```python
from build123d import *

# Parameters (mm, degrees)
SKETCH068_R         = 1
PAD021_DEPTH        = 1.3
SKETCH002_R         = 0.5
POCKET_DEPTH        = 0.001
POCKET_DEPTH_BACK   = 1.301
LINEARPATTERN_COUNT = 7
LINEARPATTERN_PITCH = 2.54


with BuildPart() as part:
    # Sketch068 → Pad021 (new body)
    with BuildSketch(Plane.XY):
        Polygon((-13.25, 19.61), (13.25, 19.61), (13.89, 18.97), (13.89, -18.97), (13.25, -19.61), (-13.25, -19.61), (-13.89, -18.97), (-13.89, 18.97), align=None)
        with Locations((11.39, 17.11)):
            Circle(SKETCH068_R, mode=Mode.SUBTRACT)
        with Locations((-11.39, 17.11)):
            Circle(SKETCH068_R, mode=Mode.SUBTRACT)
        with Locations((-11.39, -17.11)):
            Circle(SKETCH068_R, mode=Mode.SUBTRACT)
        with Locations((11.39, -17.11)):
            Circle(SKETCH068_R, mode=Mode.SUBTRACT)
    extrude(amount=PAD021_DEPTH)

    # Sketch002 → Pocket (cut, two sides)
    with BuildSketch(Plane.XY) as pocket_sk:
        with Locations((-7.62, 18.01)):
            Circle(SKETCH002_R)
    pocket = extrude(amount=-POCKET_DEPTH, mode=Mode.SUBTRACT) + extrude(pocket_sk.sketch, amount=POCKET_DEPTH_BACK, mode=Mode.SUBTRACT)

    # LinearPattern: Pocket ×7
    with Locations(*[(i * LINEARPATTERN_PITCH, 0, 0) for i in range(1, LINEARPATTERN_COUNT)]):
        add(pocket, mode=Mode.SUBTRACT)


solid = part.part
```
Verification items for the finished model (mm, model axes). Round coordinates to 2 decimals unless told otherwise and drop trailing zeros. Order: outer loops, then holes, each group sorted by start corner. A loop starts at its lowest first (then second) coordinate and runs counter-clockwise, first axis right, second up.
1) Cross-section at B-B, the plane y = 17.11. Record the cut outline in (x, z), plus the area to 3 significant figures.
Geometry says:
outline: (-13.89, 0) - (-12.39, 0) - (-12.39, 1.3) - (-13.89, 1.3) - close; (-10.39, 0) - (10.39, 0) - (10.39, 1.3) - (-10.39, 1.3) - close; (12.39, 0) - (13.89, 0) - (13.89, 1.3) - (12.39, 1.3) - close
area: 30.9 mm2
2) Draft check along Y on faces 1 (the flat face through (0, -19.61, 1)), 2 (the flat face through (-13.89, 0, 1)), 3 (the flat face through (0, 19.61, 1)), 4 (the cylindrical face through (2.81, 18.43, 0.66)). Enter one of: +Y half, -Y half, draft (parallel to the pull), parting line (faces both ways), or undercut.
Geometry says:
face 1: -Y half
face 2: draft
face 3: +Y half
face 4: undercut
3) Cross-section at A-A, the plane x = 11.39. Record the cut outline in (y, z), plus the area to 3 significant figures.
Geometry says:
outline: (-19.61, 0) - (-18.11, 0) - (-18.11, 1.3) - (-19.61, 1.3) - close; (-16.11, 0) - (16.11, 0) - (16.11, 1.3) - (-16.11, 1.3) - close; (18.11, 0) - (19.61, 0) - (19.61, 1.3) - (18.11, 1.3) - close
area: 45.8 mm2
4) Cross-section at C-C, the plane z = 0.8. Give the number of separate pieces and of enclosed holes in the cut face, plus the area to 3 significant figures.
Geometry says:
separate pieces: 1
enclosed holes: 11
area: 1,070 mm2
5) Cross-section at D-D, the plane x = -5.08. Record the cut outline in (y, z).
Geometry says:
outline: (-19.61, 0) - (17.51, 0) - (17.51, 1.3) - (-19.61, 1.3) - close; (18.51, 0) - (19.61, 0) - (19.61, 1.3) - (18.51, 1.3) - close
6) Depth check by flat-ended pin: pin 1 (2.5 mm diameter, centred on x = 11.39, y = 17.11, fed in from -Z); pin 2 (1.6 mm diameter, centred on x = 11.39, y = -17.11, fed in from -Z) (1 decimal). Enter the tip coordinate at first touch or a pass-through.
Geometry says:
pin 1: stops at z = 0
pin 2: passes through
7) Material ranges on line 1 (Y direction, x = 11.39, z = 0.85); line 2 (Y direction, x = 5, z = 0.6); line 3 (X direction, y = 17, z = 0.3), recorded low to high.
Geometry says:
line 1: y = -19.61 to -18.11, -16.11 to 16.11, 18.11 to 19.61
line 2: y = -19.61 to 17.52, 18.5 to 19.61
line 3: x = -13.89 to -12.38, -10.4 to 10.4, 12.38 to 13.89
